Build history of the part. All positions in model axes, mm. A direction names the side the tool comes from. Round coordinates to 2 decimals unless told otherwise and drop trailing zeros. Write each loop counter-clockwise with the first axis right and the second up, starting at its lowest first coordinate (ties: lowest second). Pieces come first, ordered by that corner, then holes. Notation, with made-up numbers: (-20.5, -0.5) - (27.5, -0.5) arc R37 ccw to (27.5, 35.5) - close; hole circle Ø2 at (86, 5). An arc over 180 degrees is marked (long way). Write each question's results on one line, items separated by ' | '.
from build123d import *

# Parameters (mm, degrees)
SKETCH1_R           = 28.575
SKETCH1_R_2         = 23.4315
BOSS_EXTRUDE1_DEPTH = 76.2
BOSS_EXTRUDE2_DEPTH = 76.2
BOSS_EXTRUDE4_START = -31.75
SKETCH5_R           = 12.7
BOSS_EXTRUDE4_DEPTH = 31.75
SKETCH3_R           = 23.4315
CUT_EXTRUDE1_DEPTH  = 112.487266812
SKETCH6_W           = 3.175
SKETCH6_H           = 34.556340068
CUT_EXTRUDE2_DEPTH  = 112.487266812


with BuildPart() as part:
    # Sketch1 → Boss-Extrude1 (new body)
    with BuildSketch(Plane(origin=(0, 0, 0), x_dir=(1, 0, 0), z_dir=(0, 1, 0))):
        with Locations(Location((0, 0, 0), (0, 0, 90))):
            Circle(SKETCH1_R)
        with Locations(Location((0, 0, 0), (0, 0, 90))):
            Circle(SKETCH1_R_2, mode=Mode.SUBTRACT)
    extrude(amount=BOSS_EXTRUDE1_DEPTH)

    # Sketch2 → Boss-Extrude2 (add)
    with BuildSketch(Plane.XY):
        with BuildLine():
            ThreePointArc((-6.35, 38.1), (0, 44.45), (6.35, 38.1))
            Line((6.35, 38.1), (12.7, 38.1))
            ThreePointArc((12.7, 38.1), (0, 50.8), (-12.7, 38.1))
            Line((-12.7, 38.1), (-6.35, 38.1))
        make_face()
        with BuildLine():
            Line((12.7, 38.1), (6.35, 38.1))
            ThreePointArc((6.35, 38.1), (0, 31.75), (-6.35, 38.1))
            Line((-6.35, 38.1), (-12.7, 38.1))
            ThreePointArc((-12.7, 38.1), (0, 25.4), (12.7, 38.1))
        make_face()
    extrude(amount=BOSS_EXTRUDE2_DEPTH)

    # Sketch5 → Boss-Extrude4 (add)
    with BuildSketch(Plane.XY.offset(31.75).offset(BOSS_EXTRUDE4_START)):
        with Locations(Location((0, 38.1, 0), (0, 0, 180))):
            Circle(SKETCH5_R)
    extrude(amount=BOSS_EXTRUDE4_DEPTH)

    # Sketch3 → Cut-Extrude1 (cut, through all)
    with BuildSketch(Plane(origin=(0, 76.2, 0), x_dir=(1, 0, 0), z_dir=(0, 1, 0))):
        with Locations(Location((0, 0, 0), (0, 0, 90))):
            Circle(SKETCH3_R)
    extrude(amount=-CUT_EXTRUDE1_DEPTH, mode=Mode.SUBTRACT)

    # Sketch6 → Cut-Extrude2 (cut, through all)
    with BuildSketch(Plane(origin=(0, 76.2, 0), x_dir=(1, 0, 0), z_dir=(0, 1, 0))):
        with Locations((0, 23.4315)):
            Rectangle(SKETCH6_W, SKETCH6_H)
    extrude(amount=-CUT_EXTRUDE2_DEPTH, mode=Mode.SUBTRACT)


solid = part.part
(1) Tool access for faces 4 (the flat face through (-6, 35, 76.2)), 5 (the flat face through (-1.588, 39, -26)), 6 (the cylindrical face through (6.057, 36.193, 53.664)): list every direction of +Z, -Z, +X, -X, +Y, -Y with a clear straight run to the whole face (end or side of a thin tool).
Worked answers:
face 4: +Z, +X, -X, +Y, -Y | face 5: -Z, +Y, -Y | face 6: +Z
(2) Two-plate mould, pull along X, no slides. Class faces 1 (the flat face through (1.588, 39, -26)), 2 (the flat face through (21, 76.2, 11)), 3 (the cylindrical face through (-11.732, 42.964, 50.545)): released by +X, released by -X, zero draft, split by the parting line, or undercut.
Worked answers:
face 1: undercut | face 2: zero draft | face 3: split by the parting line
(3) Slice it at D-D, the plane z = 61. Write the cut outline in (x, y), and give its area (3 significant figures).
Worked answers:
outline: circle Ø25.4 at (0, 38.1); hole circle Ø12.7 at (0, 38.1) | area: 380 mm2
(4) Slice it at A-A, the plane z = 0. Write the cut outline in (x, y) (1 decimal), and give its area (3 significant figures).
Worked answers:
outline: (-28.6, 0) - (-23.4, 0) - (-23.4, 76.2) - (-28.6, 76.2) - close; (23.4, 0) - (28.6, 0) - (28.6, 76.2) - (23.4, 76.2) - close | area: 784 mm2
(5) Flat gauge pins, fed straight in: pin 1 Ø4 at (y, z) = (51.5, 35) entering from -X; pin 2 Ø5 at (x, y) = (20.5, 41) entering from +Z; pin 3 Ø4 at (y, z) = (56.5, 24.5) entering from -X. Where does each tip first touch, or does it go through?
Worked answers:
pin 1: stops at x = -5.6 | pin 2: stops at z = 22.19 | pin 3: stops at x = -17.61
(6) Drill centre lines: probe 1 along X at (y, z) = (38, 51); probe 2 along Y at (x, z) = (0, 61); probe 3 along X at (y, z) = (49, 0) (1 decimal). Where is each one in solid material? Low to high. Write a range as [from, to].
Worked answers:
probe 1: x = [-12.7, -6.35], [6.35, 12.7] | probe 2: y = [25.4, 31.75], [44.45, 50.8] | probe 3: x = [-28.6, -23.4], [23.4, 28.6]
